from build123d import *

# Parameters (mm, degrees)
SKETCH1_R           = 2.9718
BOSS_EXTRUDE1_DEPTH = 2.3876
SKETCH2_R           = 5.9563
SKETCH2_R_2         = 2.9718
BOSS_EXTRUDE2_DEPTH = 12.7
SKETCH3_R           = 2.9718
BOSS_EXTRUDE3_DEPTH = 2.3876


with BuildPart() as part:
    # Sketch1 → Boss-Extrude1 (new body)
    # profile 1 of 7: a face of its own
    with BuildSketch(Plane.XY):
        with BuildLine():
            Line((-5.02285, 4.50215), (-9.525, 9.0043))
            ThreePointArc((-9.525, 9.0043), (-18.3562849, -1.756651787), (-6.07920357, -8.318888475))
            ThreePointArc((-6.07920357, -8.318888475), (-6.038523344, -8.30173624), (-5.997794724, -8.284699236))
            ThreePointArc((-5.997794724, -8.284699236), (-2.013760656, -4.965752915), (-0.5207, 0))
            Line((-0.5207, 0), (-5.02285, 4.50215))
        make_face()
        with Locations((-9.525, 0)):
            Circle(SKETCH1_R, mode=Mode.SUBTRACT)
    # profile 2 of 7: a face of its own
    with BuildSketch(Plane.XY):
        with BuildLine():
            ThreePointArc((-6.07920357, 8.318888475), (-7.768348213, 8.8312849), (-9.525, 9.0043))
            Line((-9.525, 9.0043), (-5.02285, 4.50215))
            Line((-5.02285, 4.50215), (-3.15799841, 6.36700159))
            ThreePointArc((-3.15799841, 6.36700159), (-4.485831076, 7.462184335), (-5.997794724, 8.284699236))
            ThreePointArc((-5.997794724, 8.284699236), (-6.038523344, 8.30173624), (-6.07920357, 8.318888475))
        make_face()
    # profile 3 of 7: a face of its own
    with BuildSketch(Plane.XY):
        with BuildLine():
            ThreePointArc((-3.15799841, 6.36700159), (-1.206111525, 3.44579643), (-0.5207, 0))
            ThreePointArc((-0.5207, 0), (-2.013760656, -4.965752915), (-5.997794724, -8.284699236))
            ThreePointArc((-5.997794724, -8.284699236), (0, -7.08520242), (5.997794724, -8.284699236))
            ThreePointArc((5.997794724, -8.284699236), (0.685208337, -1.713330628), (3.15799841, 6.36700159))
            Line((3.15799841, 6.36700159), (0, 6.36700159))
            Line((0, 6.36700159), (-3.15799841, 6.36700159))
        make_face()
    # profile 4 of 7: a face of its own
    with BuildSketch(Plane.XY):
        with BuildLine():
            Line((-3.15799841, 6.36700159), (-5.02285, 4.50215))
            Line((-5.02285, 4.50215), (-0.5207, 0))
            ThreePointArc((-0.5207, 0), (-1.206111525, 3.44579643), (-3.15799841, 6.36700159))
        make_face()
    # profile 5 of 7: a face of its own
    with BuildSketch(Plane.XY):
        with BuildLine():
            ThreePointArc((-5.997794724, 8.284699236), (-4.485831076, 7.462184335), (-3.15799841, 6.36700159))
            Line((-3.15799841, 6.36700159), (0, 6.36700159))
            Line((0, 6.36700159), (0, 7.08520242))
            ThreePointArc((0, 7.08520242), (-3.058281141, 7.388016551), (-5.997794724, 8.284699236))
        make_face()
    # profile 6 of 7: a face of its own
    with BuildSketch(Plane.XY):
        with BuildLine():
            ThreePointArc((5.997794724, 8.284699236), (3.058281141, 7.388016551), (0, 7.08520242))
            Line((0, 7.08520242), (0, 6.36700159))
            Line((0, 6.36700159), (3.15799841, 6.36700159))
            ThreePointArc((3.15799841, 6.36700159), (4.485831076, 7.462184335), (5.997794724, 8.284699236))
        make_face()
    # profile 7 of 7: a face of its own
    with BuildSketch(Plane.XY):
        with BuildLine():
            ThreePointArc((18.5293, 0), (15.89200159, 6.36700159), (9.525, 9.0043))
            ThreePointArc((9.525, 9.0043), (7.768348213, 8.8312849), (6.07920357, 8.318888475))
            ThreePointArc((6.07920357, 8.318888475), (6.038523344, 8.30173624), (5.997794724, 8.284699236))
            ThreePointArc((5.997794724, 8.284699236), (4.485831076, 7.462184335), (3.15799841, 6.36700159))
            ThreePointArc((3.15799841, 6.36700159), (0.685208337, -1.713330628), (5.997794724, -8.284699236))
            ThreePointArc((5.997794724, -8.284699236), (6.038523344, -8.30173624), (6.07920357, -8.318888475))
            ThreePointArc((6.07920357, -8.318888475), (14.527521049, -7.48680183), (18.5293, 0))
        make_face()
        with Locations((9.525, 0)):
            Circle(SKETCH1_R, mode=Mode.SUBTRACT)
    extrude(amount=BOSS_EXTRUDE1_DEPTH)

    # Sketch2 → Boss-Extrude2 (add)
    # profile 1 of 2: a face of its own
    with BuildSketch(Plane.XY.offset(2.3876)):
        with Locations((9.525, 0)):
            Circle(SKETCH2_R)
        with Locations((9.525, 0)):
            Circle(SKETCH2_R_2, mode=Mode.SUBTRACT)
    # profile 2 of 2: a face of its own
    with BuildSketch(Plane.XY.offset(2.3876)):
        with Locations((-9.525, 0)):
            Circle(SKETCH2_R)
        with Locations((-9.525, 0)):
            Circle(SKETCH2_R_2, mode=Mode.SUBTRACT)
    extrude(amount=BOSS_EXTRUDE2_DEPTH)

    # Sketch3 → Boss-Extrude3 (add)
    with BuildSketch(Plane.XY.offset(15.0876)):
        with BuildLine():
            ThreePointArc((6.07920357, -8.318888475), (18.5293, 0), (6.07920357, 8.318888475))
            ThreePointArc((6.07920357, 8.318888475), (0, 7.08520242), (-6.07920357, 8.318888475))
            ThreePointArc((-6.07920357, 8.318888475), (-18.5293, 0), (-6.07920357, -8.318888475))
            ThreePointArc((-6.07920357, -8.318888475), (0, -7.08520242), (6.07920357, -8.318888475))
        make_face()
        with Locations((-9.525, 0)):
            Circle(SKETCH3_R, mode=Mode.SUBTRACT)
        with Locations((9.525, 0)):
            Circle(SKETCH3_R, mode=Mode.SUBTRACT)
    extrude(amount=BOSS_EXTRUDE3_DEPTH)


solid = part.part
CAD build for the part. Positions are in the model's coordinates, mm. A direction names the side the tool comes from. Round coordinates to 2 decimals unless told otherwise and drop trailing zeros. Order: outer loops, then holes, each group sorted by start corner. A loop starts at its lowest first (then second) coordinate and runs counter-clockwise, first axis right, second up. Notation, with made-up numbers: (85, 28.5) - (111, 28.5) arc R19 cw to (111, 62.5) - close; hole circle Ø4 at (-36, -38.75). An arc over 180 degrees is marked (long way). Return JSON: item names as keys, results as strings.
(1) Cut at D-D (z = 16). Give the cut face in (x, y) (3 decimals), then the cut area to 3 significant figures.
Answer key:
{"outline": "(-6.079, -8.319) arc R15.595 cw to (6.079, -8.319) arc R9.004 ccw (long way) to (6.079, 8.319) arc R15.595 cw to (-6.079, 8.319) arc R9.004 ccw (long way) to start; hole circle Ø5.944 at (-9.525, 0); hole circle Ø5.944 at (9.525, 0)", "area": "502 mm^2"}
(2) Pin check, flat tips, straight feed: pin 1 Ø1 at (y, z) = (-2, 11) entering from +X; pin 2 Ø3 at (x, z) = (-13, 6.5) entering from +Y; pin 3 Ø2 at (y, z) = (0.5, 15) entering from +X; pin 4 Ø1 at (y, z) = (-6, 11) entering from -X. Stop position of each tip, or through.
Answer key:
{"pin 1": "stops at x = 15.29", "pin 2": "stops at y = 5.62", "pin 3": "stops at x = 18.53", "pin 4": "stops at x = -11.81"}
(3) Cut at B-B (x = 7). Give the cut face in (y, z).
Answer key:
{"outline": "(-8.64, 0) - (-1.57, 0) - (-1.57, 17.48) - (-8.64, 17.48) - (-8.64, 15.09) - (-5.39, 15.09) - (-5.39, 2.39) - (-8.64, 2.39) - close; (1.57, 0) - (8.64, 0) - (8.64, 2.39) - (5.39, 2.39) - (5.39, 15.09) - (8.64, 15.09) - (8.64, 17.48) - (1.57, 17.48) - close"}
(4) Pull direction Y, two halves, no side cores. Call faces 3 (the face through (-0.086, -7.085, 1.177)), 4 (the face through (-12.494, 0.131, 8.615)), 5 (the face through (0, 0, 2.388)): +Y half, -Y half, draft (parallel to the pull), parting line (faces both ways), or undercut.
Answer key:
{"face 3": "-Y half", "face 4": "undercut", "face 5": "draft"}
(5) Tool access for faces 1 (the face through (0, 0, 0)), 2 (the face through (0, 0, 15.088)): list every direction of +Z, -Z, +X, -X, +Y, -Y with a clear straight run to the whole face (end or side of a thin tool).
Answer key:
{"face 1": "-Z, +X, -X, +Y, -Y", "face 2": "none"}
(6) Cut at A-A (y = 2.5). Give the cut face in (x, z), then the cut area to 3 significant figures.
Answer key:
{"outline": "(-18.18, 0) - (-11.13, 0) - (-11.13, 17.48) - (-18.18, 17.48) - (-18.18, 15.09) - (-14.93, 15.09) - (-14.93, 2.39) - (-18.18, 2.39) - close; (-7.92, 0) - (7.92, 0) - (7.92, 17.48) - (-7.92, 17.48) - close; (11.13, 0) - (18.18, 0) - (18.18, 2.39) - (14.93, 2.39) - (14.93, 15.09) - (18.18, 15.09) - (18.18, 17.48) - (11.13, 17.48) - close; hole (-4.12, 2.39) - (4.12, 2.39) - (4.12, 15.09) - (-4.12, 15.09) - close", "area": "336 mm^2"}
(7) Wall check: probe 1 along Z at (x, y) = (-7, -6.75); probe 2 along X at (y, z) = (-0.5, 7.75); probe 3 along Y at (x, z) = (-0.5, 2.25). Give the ranges that are in metal, low to high. Write a range as from..to.
Answer key:
{"probe 1": "z = 0..2.39, 15.09..17.48", "probe 2": "x = -15.46..-12.45, -6.6..-3.59, 3.59..6.6, 12.45..15.46", "probe 3": "y = -7.09..7.09"}
(8) Cut at C-C (z = 3.5). Give the cut face in (x, y) (3 decimals), then the cut area to 3 significant figures.
Answer key:
{"outline": "circle Ø11.913 at (-9.525, 0); circle Ø11.913 at (9.525, 0); hole circle Ø5.944 at (-9.525, 0); hole circle Ø5.944 at (9.525, 0)", "area": "167 mm^2"}
